```python
from build123d import *


with BuildPart() as part:
    # Sweep1: sweep along a curve in space
    with BuildLine() as sweep1_path:
        add(Edge.make_bspline(
            [(0, 28.600823045, -25), (515.519545798, 52.9249772, -25), (1099.508665119, 21.327347601, -25)],
            knots=[0, 0, 0, 1, 1, 1], degree=2))
    # Sketch2 → Sweep1 (sweep)
    with BuildSketch(Plane(origin=(0, 0, 0), x_dir=(0, 0, -1), z_dir=(1, 0, 0))):
        with BuildLine():
            Line((0, 48.148148148), (50, 48.148148148))
            ThreePointArc((50, 48.148148148), (69.547325103, 28.600823045), (50, 9.053497942))
            Line((50, 9.053497942), (0, 9.053497942))
            ThreePointArc((0, 9.053497942), (-19.547325103, 28.600823045), (0, 48.148148148))
        make_face()
    sweep(path=sweep1_path.line)

    # Cut-Sweep1: sweep along a curve in space
    with BuildLine() as cut_sweep1_path:
        add(Edge.make_bspline(
            [(0, 28.600823045, -25), (515.519545798, 52.9249772, -25), (1099.508665119, 21.327347601, -25)],
            knots=[0, 0, 0, 1, 1, 1], degree=2))
    # Sketch3 → Cut-Sweep1 (sweep, cut)
    with BuildSketch(Plane.ZY):
        Polygon((-40, 19.053497942), (-10, 19.053497942), (-10, 14.053497942), (-22.5, 14.053497942), (-22.5, 9.053497942), (-22.174756388, 5.22639824), (-27.5, 5.22639824), (-27.5, 9.053497942), (-27.5, 14.053497942), (-40, 14.053497942), align=None)
    sweep(path=cut_sweep1_path.line, mode=Mode.SUBTRACT)


solid = part.part
```
The model under review builds one solid part; all positions refer to its coordinate system, in mm. A direction names the side the tool comes from. Coordinates: 2 decimals unless noted, no trailing zeros. One line per item, written item: value. Start each with the question number.
Q1. For faces 1 (the face through (511, 20, -22.5)), 2 (the face through (1099.48, 21.06, -24.3)), 3 (the face through (511, 25, -10)), list the 3-axis set-ups (+Z, -Z, +X, -X, +Y, -Y) from which the entire face can be reached by the end or side of a thin tool; tool diameter is ignored.
Q2. To check wall thickness, follow probe 1 along Z at (x, y) = (355, 40); probe 2 along Z at (x, y) = (167.5, 19); probe 3 along Y at (x, z) = (226.5, -15). State the ranges of each line that lie inside material, in increasing order.
Q3. Clearance check with flat-ended pins moving along their axes: P1, Ø4, axis at x = 573, y = 34.5, coming from the +Z side; P2, Ø6, axis at x = 715.5, z = 7, coming from the +Y side; P3, Ø2, axis at x = 824.5, z = -57, coming from the +Y side; P4, Ø1.5, axis at x = 179, y = 14, coming from the +Z side. State where each tip first meets the part, or that it passes through.
Q4. The part is to be moulded in two halves that separate along Z. For faces 4 (the face through (0, 28, -24)), 5 (the face through (551.6, 19.5, -27.5)), say which applies: +Z half, -Z half, draft (parallel to the pull), parting line (faces both ways), or undercut.
Response:
1. face 1: -Y
1. face 2: +Z, -Z, +X, -Y
1. face 3: none
2. probe 1: -69.5 to 19.5
2. probe 2: -61.25 to -27.5, -22.5 to 11.25
2. probe 3: 16.98 to 21.98, 26.97 to 56.04
3. P1: z = 19.43
3. P2: y = 55.35
3. P3: y = 51.82
3. P4: through
4. face 4: draft
4. face 5: undercut
